Can you work these out from the model? Positions are in its coordinate system, mm. A direction names the side the tool comes from. Coordinates: 2 decimals unless noted, no trailing zeros. Order: outer loops, then holes, each group sorted by start corner. A loop starts at its lowest first (then second) coordinate and runs counter-clockwise, first axis right, second up. Notation, with made-up numbers: (84, -32.75) -> (128, -32.75) arc R16 cw to (128, -3.75) -> close; hole circle Ø4 at (87.5, -38). An arc over 180 degrees is marked (long way). Use a Markdown table: item, result. Add a question column.
1. Suppose I cut it at A-A, the plane z = 34. List the corners of the cut face in (x, y) for me, then the cut area to 3 significant figures.
2. Suppose I cut it at C-C, the plane y = -4. List the corners of the cut face in (x, z) for me.
3. If I drill on line 1 along X through (y, z) = (-12, 13); line 2 along Z through (x, y) = (4, -15), over which ranges is the centre line in solid material (lowest first)? Write a range as from..to.
4. For pin 1 Ø1.5 at (y, z) = (-9, 14) entering from +X; pin 2 Ø8 at (x, z) = (20.5, 8) entering from +Y; pin 3 Ø5 at (y, z) = (-10.5, 4) entering from +X, each with a flat end and sliding along its axis, tell me the tip position at first contact or that it passes through.
5. Suppose I cut it at B-B, the plane x = -5.5. List the corners of the cut face in (y, z) for me, then the cut area to 3 significant figures.
6. For faces 1 (the flat face through (29, -25, 19)), 2 (the flat face through (-21, 4, 23)), which set-ups out of +Z, -Z, +X, -X, +Y, -Y let a thin tool reach every point of the face, with its end or its side?
```python
from build123d import *

# Parameters (mm, degrees)
F0_W     = 58
F0_H     = 58
F1_DEPTH = 8
F3_DEPTH = 30
F5_DEPTH = 8.001
F6_R     = 5


with BuildPart() as f1:
    # F0 (on Top) → F1 (new body)
    with BuildSketch(Plane.XY):
        Rectangle(F0_W, F0_H)
    extrude(amount=F1_DEPTH)

    # F2 (on face) → F3 (join)
    with BuildSketch(Plane.XY.offset(8)):
        Polygon((-29, 29), (-29, -29), (29, -29), (29, -21), (-21, -21), (-21, 29), align=None)
    extrude(amount=F3_DEPTH)

    # F4 (on face) → F5 (cut, through all)
    with BuildSketch(Plane.XY.offset(8)):
        Polygon((29, 29), (-21, 29), (29, -21), align=None)
    extrude(amount=-F5_DEPTH, mode=Mode.SUBTRACT)

    # F6
    f6_edges = [f1.edges().sort_by_distance(p)[0] for p in [
        (-29, -29, 19),
    ]]
    fillet(f6_edges, radius=F6_R)


solid = f1.part
```
Worked out:
| question | item | result |
|---|---|---|
| 1 | outline | (-29, -24) arc R5 ccw to (-24, -29) -> (29, -29) -> (29, -21) -> (-21, -21) -> (-21, 29) -> (-29, 29) -> close |
| 1 | area | 859 mm² |
| 2 | outline | (-29, 0) -> (12, 0) -> (12, 8) -> (-21, 8) -> (-21, 38) -> (-29, 38) -> close |
| 3 | line 1 | x = -29..-21 |
| 3 | line 2 | z = 0..8 |
| 4 | pin 1 | stops at x = -21 |
| 4 | pin 2 | stops at y = -8.5 |
| 4 | pin 3 | stops at x = 21 |
| 5 | outline | (-29, 0) -> (13.5, 0) -> (13.5, 8) -> (-21, 8) -> (-21, 38) -> (-29, 38) -> close |
| 5 | area | 580 mm² |
| 6 | face 1 | +Z, -Z, +X, +Y, -Y |
| 6 | face 2 | +Z, +X, +Y |
